```python
from build123d import *

# Parameters (mm, degrees)
SKETCH1_W           = 76.2
SKETCH1_H           = 76.2
BOSS_EXTRUDE1_DEPTH = 38.1
SKETCH2_OUTSIDE_W   = 101.06
SKETCH2_OUTSIDE_H   = 101.06
CUT_EXTRUDE1_DEPTH  = 66.991135768
CUT_EXTRUDE2_DEPTH  = 38.1
CUT_EXTRUDE3_DEPTH  = 38.1


with BuildPart() as part:
    # Sketch1 → Boss-Extrude1 (new body)
    with BuildSketch(Plane(origin=(0, 0, 0), x_dir=(1, 0, 0), z_dir=(0, 1, 0))):
        Rectangle(SKETCH1_W, SKETCH1_H)
    extrude(amount=BOSS_EXTRUDE1_DEPTH)

    # Sketch2 outside → Cut-Extrude1 (cut, through all)
    with BuildSketch(Plane(origin=(0, 38.1, 0), x_dir=(1, 0, 0), z_dir=(0, 1, 0))):
        Rectangle(SKETCH2_OUTSIDE_W, SKETCH2_OUTSIDE_H)
        Polygon((-38.1, 38.1), (38.1, 38.1), (38.1, 31.75), (38.1, -38.1), (31.75, -38.1), (31.75, 31.75), (-38.1, 31.75), align=None, mode=Mode.SUBTRACT)
    extrude(amount=-CUT_EXTRUDE1_DEPTH, mode=Mode.SUBTRACT)

    # Sketch4 → Cut-Extrude2 (cut)
    with BuildSketch(Plane.XY.offset(-31.75)):
        with BuildLine():
            Line((-25.908, 19.05), (-22.225, 19.05))
            Line((-22.225, 19.05), (-18.542, 19.05))
            ThreePointArc((-18.542, 19.05), (-22.225, 22.733), (-25.908, 19.05))
        make_face()
        with BuildLine():
            Line((-18.542, 19.05), (-22.225, 19.05))
            Line((-22.225, 19.05), (-25.908, 19.05))
            ThreePointArc((-25.908, 19.05), (-22.225, 15.367), (-18.542, 19.05))
        make_face()
        with BuildLine():
            ThreePointArc((19.558, 19.05), (15.875, 22.733), (12.192, 19.05))
            Line((12.192, 19.05), (15.875, 19.05))
            Line((15.875, 19.05), (19.558, 19.05))
        make_face()
        with BuildLine():
            Line((15.875, 19.05), (12.192, 19.05))
            ThreePointArc((12.192, 19.05), (15.875, 15.367), (19.558, 19.05))
            Line((19.558, 19.05), (15.875, 19.05))
        make_face()
    extrude(amount=-CUT_EXTRUDE2_DEPTH, mode=Mode.SUBTRACT)

    # Sketch5 → Cut-Extrude3 (cut)
    with BuildSketch(Plane.ZY.offset(-31.75)):
        with BuildLine():
            Line((-19.558, 19.05), (-15.875, 19.05))
            Line((-15.875, 19.05), (-12.192, 19.05))
            ThreePointArc((-12.192, 19.05), (-15.875, 22.733), (-19.558, 19.05))
        make_face()
        with BuildLine():
            Line((-12.192, 19.05), (-15.875, 19.05))
            Line((-15.875, 19.05), (-19.558, 19.05))
            ThreePointArc((-19.558, 19.05), (-15.875, 15.367), (-12.192, 19.05))
        make_face()
        with BuildLine():
            ThreePointArc((25.908, 19.05), (22.225, 22.733), (18.542, 19.05))
            Line((18.542, 19.05), (22.225, 19.05))
            Line((22.225, 19.05), (25.908, 19.05))
        make_face()
        with BuildLine():
            Line((22.225, 19.05), (18.542, 19.05))
            ThreePointArc((18.542, 19.05), (22.225, 15.367), (25.908, 19.05))
            Line((25.908, 19.05), (22.225, 19.05))
        make_face()
    extrude(amount=-CUT_EXTRUDE3_DEPTH, mode=Mode.SUBTRACT)


solid = part.part
```
Geometry: final body of the model. Coordinates: model frame, mm. A direction names the side the tool comes from. Coordinates: 2 decimals unless noted, no trailing zeros. Loops run counter-clockwise (first coordinate to the right, second up) from the corner with the lowest first, then second, coordinate; pieces in that order, holes last. Notation, with made-up numbers: (-25.5, 51.5) -> (6.5, 51.5) arc R35 cw to (6.5, 83.5) -> close; hole circle Ø11 at (73, -14.75). An arc over 180 degrees is marked (long way). Use a Markdown table: item, result. Add a question column.
(1) Section query B-B, the plane y = 26. Return loops of the section in (x, z).
(2) Section query A-A, the plane y = 19.05. Return loops of the section in (x, z).
(3) Pin query (flat end, axial travel): pin 1 Ø12 at (y, z) = (19.05, -15.875) entering from -X; pin 2 Ø10 at (x, y) = (-17, 4.5) entering from +Z. Return the tip coordinate at first contact, or that it passes through.
(4) Access query for faces 4 (the flat face through (17, 0, -34)), 5 (the flat face through (-3, 19, -31.75)). Directions: +Z, -Z, +X, -X, +Y, -Y. A direction counts if a zero-diameter tool reaches every point of the face in a straight line with its end or side. Return the directions, or none.
(5) Line query: line 1 along Z through (x, y) = (35, 19.05); line 2 along X through (y, z) = (5, 25.5); line 3 along Z through (x, y) = (-18, 2). Output: solid intervals per line, ascending.
(6) Section query C-C, the plane x = 28.5. Return loops of the section in (y, z), plus the area to 3 significant figures.
(7) Section query D-D, the plane z = 8. Return loops of the section in (x, y).
(8) Mould query, pull axis Z, two halves, no side actions, for faces 1 (the flat face through (35, 19, 38.1)), 2 (the cylindrical face through (34.88, 15.94, 20.25)), 3 (the flat face through (17, 38.1, -34)). Classes: pulls with the +Z half, pulls with the -Z half, needs draft (parallel to the pull), parting line crosses it, or undercut.
Answer:
| question | item | result |
|---|---|---|
| 1 | outline | (-38.1, -38.1) -> (38.1, -38.1) -> (38.1, 38.1) -> (31.75, 38.1) -> (31.75, -31.75) -> (-38.1, -31.75) -> close |
| 2 | outline | (-38.1, -38.1) -> (-25.91, -38.1) -> (-25.91, -31.75) -> (-38.1, -31.75) -> close; (-18.54, -38.1) -> (12.19, -38.1) -> (12.19, -31.75) -> (-18.54, -31.75) -> close; (19.56, -38.1) -> (38.1, -38.1) -> (38.1, -19.56) -> (31.75, -19.56) -> (31.75, -31.75) -> (19.56, -31.75) -> close; (31.75, -12.19) -> (38.1, -12.19) -> (38.1, 18.54) -> (31.75, 18.54) -> close; (31.75, 25.91) -> (38.1, 25.91) -> (38.1, 38.1) -> (31.75, 38.1) -> close |
| 3 | pin 1 | stops at x = 31.75 |
| 3 | pin 2 | stops at z = -31.75 |
| 4 | face 4 | +Z, -Z, +X, -X, -Y |
| 4 | face 5 | +Z, -X, +Y, -Y |
| 5 | line 1 | z = -38.1 to -19.56, -12.19 to 18.54, 25.91 to 38.1 |
| 5 | line 2 | x = 31.75 to 38.1 |
| 5 | line 3 | z = -38.1 to -31.75 |
| 6 | outline | (0, -38.1) -> (38.1, -38.1) -> (38.1, -31.75) -> (0, -31.75) -> close |
| 6 | area | 242 mm^2 |
| 7 | outline | (31.75, 0) -> (38.1, 0) -> (38.1, 38.1) -> (31.75, 38.1) -> close |
| 8 | face 1 | pulls with the +Z half |
| 8 | face 2 | undercut |
| 8 | face 3 | needs draft |
